Geometry: final body of the model. Coordinates: model frame, mm. Face numbers are marked on the shaded views. Give positions to 0.01 mm unless a question says otherwise; leave off trailing zeros. Loops run counter-clockwise (first coordinate to the right, second up) from the corner with the lowest first, then second, coordinate; pieces in that order, holes last.
1. First-contact query: P1, Ø2.5, axis at x = -30, y = -1.323, coming from the +Z side; P2, Ø1.7, axis at x = 4, z = 7.5, coming from the -Y side; P3, Ø6, axis at x = 2, y = -3.5, coming from the +Z side. Flat tips, straight axial feed; report the tip coordinate or a pass-through.
2. Section A-A, the plane x = 30. Output: boundary loops of the cut face in (y, z).
3. Section C-C, the plane y = 2.25. Output: boundary loops of the cut face in (x, z), then the cut area to 3 significant figures.
4. Section B-B, the plane z = 4.5. Output: boundary loops of the cut face in (x, y), then the cut area to 3 significant figures.
5. Draft query along X for the marked faces 1, 2 and 3. Return one class per face: +X half, -X half, draft (parallel to the pull), parting line (faces both ways), or undercut.
6. Material intervals for line 1 along X through (y, z) = (-1.5, 4); line 2 along Y through (x, z) = (30, 5.5); line 3 along X through (y, z) = (-4, 6), sorted ascending.
7. Section D-D, the plane x = -10. Output: boundary loops of the cut face in (y, z).
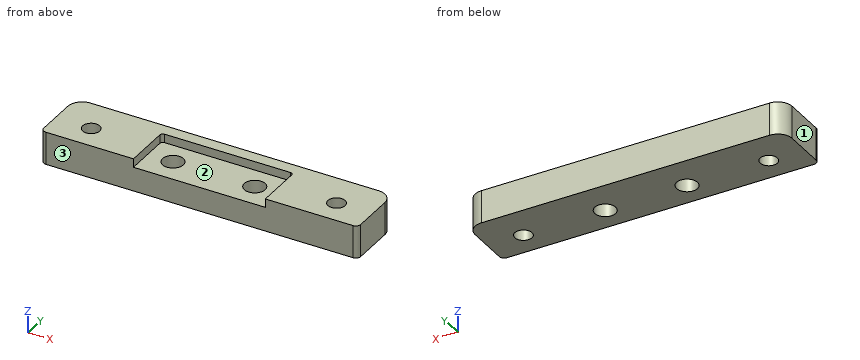
from build123d import *

# Parameters (mm, degrees)
SKETCH1_W             = 77.5
SKETCH1_H             = 14.874
BOSS_EXTRUDE1_DEPTH   = 8
SKETCH2_W             = 32.24
SKETCH2_H             = 11.877
CUT_EXTRUDE1_DEPTH    = 2.1
FILLET1_R             = 3.5
FILLET2_R             = 0.75
SKETCH3_R             = 2.55
CUT_EXTRUDE2_DEPTH    = 6.9
M5X0_8_TAPPED_HOLE1_D = 4.2
FILLET3_R             = 1.2


with BuildPart() as part:
    # Sketch1 → Boss-Extrude1 (new body)
    with BuildSketch(Plane.XY):
        Rectangle(SKETCH1_W, SKETCH1_H)
    extrude(amount=BOSS_EXTRUDE1_DEPTH)

    # Sketch2 → Cut-Extrude1 (cut)
    with BuildSketch(Plane.XY.offset(8)):
        with Locations((0, -1.4985)):
            Rectangle(SKETCH2_W, SKETCH2_H)
    extrude(amount=-CUT_EXTRUDE1_DEPTH, mode=Mode.SUBTRACT)

    # Fillet1
    fillet1_edges = [part.edges().sort_by_distance(p)[0] for p in [
        (-38.75, 7.437, 4),
        (38.75, 7.437, 4),
    ]]
    fillet(fillet1_edges, radius=FILLET1_R)

    # Fillet2
    fillet2_edges = [part.edges().sort_by_distance(p)[0] for p in [
        (-16.12, 4.44, 6.95),
        (16.12, 4.44, 6.95),
    ]]
    fillet(fillet2_edges, radius=FILLET2_R)

    # Sketch3 → Cut-Extrude2 (cut, through all)
    with BuildSketch(Plane.XY.offset(5.9)):
        with Locations((-10, -1.323)):
            Circle(SKETCH3_R)
        with Locations((10, -1.323)):
            Circle(SKETCH3_R)
    extrude(amount=-CUT_EXTRUDE2_DEPTH, mode=Mode.SUBTRACT)

    # M5x0.8 Tapped Hole1 (through all)
    with Locations(Plane.XY.offset(8)):
        with Locations((-30, -1.323), (30, -1.323)):
            Hole(M5X0_8_TAPPED_HOLE1_D / 2)

    # Fillet3
    fillet3_edges = [part.edges().sort_by_distance(p)[0] for p in [
        (38.75, -7.437, 4),
        (-38.75, -7.437, 4),
    ]]
    fillet(fillet3_edges, radius=FILLET3_R)


solid = part.part
Answers below:
1. P1: passes through
1. P2: stops at y = 4.44
1. P3: stops at z = 5.9
2. outline: (-7.44, 0) - (-3.42, 0) - (-3.42, 8) - (-7.44, 8) - close; (0.78, 0) - (7.44, 0) - (7.44, 8) - (0.78, 8) - close
3. outline: (-38.75, 0) - (38.75, 0) - (38.75, 8) - (16.12, 8) - (16.12, 5.9) - (-16.12, 5.9) - (-16.12, 8) - (-38.75, 8) - close
3. area: 552 mm2
4. outline: (-38.75, -6.24) arc R1.2 ccw to (-37.55, -7.44) - (37.55, -7.44) arc R1.2 ccw to (38.75, -6.24) - (38.75, 3.94) arc R3.5 ccw to (35.25, 7.44) - (-35.25, 7.44) arc R3.5 ccw to (-38.75, 3.94) - close; hole circle Ø4.2 at (-30, -1.32); hole circle Ø5.1 at (-10, -1.32); hole circle Ø5.1 at (10, -1.32); hole circle Ø4.2 at (30, -1.32)
4. area: 1,080 mm2
5. face 1: -X half
5. face 2: undercut
5. face 3: draft
6. line 1: x = -38.75 to -32.09, -27.91 to -12.54, -7.46 to 7.46, 12.54 to 27.91, 32.09 to 38.75
6. line 2: y = -7.44 to -3.42, 0.78 to 7.44
6. line 3: x = -38.75 to -16.12, 16.12 to 38.75
7. outline: (-7.44, 0) - (-3.87, 0) - (-3.87, 5.9) - (-7.44, 5.9) - close; (1.23, 0) - (7.44, 0) - (7.44, 8) - (4.44, 8) - (4.44, 5.9) - (1.23, 5.9) - close
